Check sheet for the modelled part. Datum: model origin and axes. Units: mm. A direction names the side the tool comes from. Give positions to 0.01 mm unless a question says otherwise; leave off trailing zeros. Order: outer loops, then holes, each group sorted by start corner. A loop starts at its lowest first (then second) coordinate and runs counter-clockwise, first axis right, second up. Notation, with made-up numbers: M 2.5,42.5 L 14.5,42.5 A25 cw 14.5,81.5 Z; hole C 19,12 d4. An arc over 180 degrees is marked long. Answer in a Markdown table with one row per item. Add a question column.
from build123d import *

# Parameters (mm, degrees)
F1_DEPTH = 79.375
F3_D     = 15.875
F3_DEPTH = 50.8
F3_TIP   = 4.7693311635
F5_D     = 6.5278
F5_DEPTH = 23.2833333333
F5_TIP   = 1.9611489744


with BuildPart() as f1:
    # F0 (on Right) → F1 (new body, symmetric)
    with BuildSketch(Plane.YZ):
        Polygon((-60.325, 63.5), (-60.325, -63.5), (60.325, -63.5), (60.325, 3.175), (0, 63.5), align=None)
    extrude(amount=F1_DEPTH, both=True)

    # F3
    with Locations(Plane.XZ.offset(60.325)):
        with Locations((-40.3225, -42.8625), (-40.3225, 33.4772), (38.1508, 33.4772)):
            Hole(F3_D / 2, depth=F3_DEPTH)
            with Locations((0, 0, -(F3_DEPTH + F3_TIP / 2))):  # 118° drill point
                Cone(0, F3_D / 2, F3_TIP, mode=Mode.SUBTRACT)

    # F5
    with Locations(Plane.YZ.offset(79.375)):
        with Locations((-44.069, 43.307), (-44.069, -1.905), (-12.319, -1.905), (-12.319, 43.307)):
            Hole(F5_D / 2, depth=F5_DEPTH)
            with Locations((0, 0, -(F5_DEPTH + F5_TIP / 2))):  # 118° drill point
                Cone(0, F5_D / 2, F5_TIP, mode=Mode.SUBTRACT)


solid = f1.part
Q1. Cross-section at C-C (y = -38). Record the boundary of the cut face in (x, z) (1 decimal).
Q2. Cross-section at A-A (x = 6.5). Record the boundary of the cut face in (y, z) (3 decimals), and give its area (3 significant figures).
Q3. Cross-section at D-D (y = 49). Record the boundary of the cut face in (x, z) (3 decimals).
Q4. Cross-section at B-B (z = 18.5). Record the boundary of the cut face in (x, y) (3 decimals).
Q5. Draft check along X on faces 1 (the cylindrical face through (67.57, -47.18, -0.92)), 2 (the conical face through (54.47, -43.53, -1.73)), 3 (the conical face through (-39.049, -5.584, -43.39)). Enter one of: pulls with the +X half, pulls with the -X half, needs draft (parallel to the pull), parting line crosses it, or undercut.
Q6. Thickness scan on probe 1 along X at (y, z) = (-28.5, 38) (3 decimals); probe 2 along X at (y, z) = (-53.5, 30.5) (1 decimal); probe 3 along Y at (x, z) = (57, -3.5) (3 decimals). Record the ranges inside material, lowest first.
Q7. Go/stop test with flat-tipped pins: pin 1 (1 mm diameter, centred on x = -45.5, z = 31, fed in from -Y); pin 2 (18.5 mm diameter, centred on x = 38.15, z = 33.48, fed in from +Y); pin 3 (10 mm diameter, centred on x = 10, z = 15, fed in from +Y). Record where each tip stops, or that it passes through.
Q8. Tool access check on faces 4 (the cylindrical face through (67.57, -9.06, -1.76)), 5 (the cylindrical face through (-38.6, -34.57, -50.61)), 6 (the flat face through (1, -1, -63.5)). Record the directions out of +Z, -Z, +X, -X, +Y, -Y that give a thin tool (end or side, any length) a straight path to the whole face; none if there is none.
Values follow:
| question | item | result |
|---|---|---|
| 1 | outline | M -79.4,-63.5 L 79.4,-63.5 L 79.4,63.5 L -79.4,63.5 Z; hole C -40.3,-42.9 d15.9; hole C -40.3,33.5 d15.9; hole C 38.2,33.5 d15.9 |
| 2 | outline | M -60.325,-63.5 L 60.325,-63.5 L 60.325,3.175 L 0,63.5 L -60.325,63.5 Z |
| 2 | area | 13,500 mm² |
| 3 | outline | M -79.375,-63.5 L 79.375,-63.5 L 79.375,14.5 L -79.375,14.5 Z |
| 4 | outline | M -79.375,-60.325 L 79.375,-60.325 L 79.375,45 L -79.375,45 Z |
| 5 | face 1 | needs draft |
| 5 | face 2 | pulls with the +X half |
| 5 | face 3 | undercut |
| 6 | probe 1 | -79.375 to -46.845, -33.8 to 31.628, 44.674 to 79.375 |
| 6 | probe 2 | -79.4 to -47.7, -33 to 30.8, 45.5 to 79.4 |
| 6 | probe 3 | -60.325 to -46.917, -41.221 to -15.167, -9.471 to 60.325 |
| 7 | pin 1 | y = -8.5 |
| 7 | pin 2 | y = 39.27 |
| 7 | pin 3 | y = 53.5 |
| 8 | face 4 | +X |
| 8 | face 5 | -Y |
| 8 | face 6 | -Z, +X, -X, +Y, -Y |
